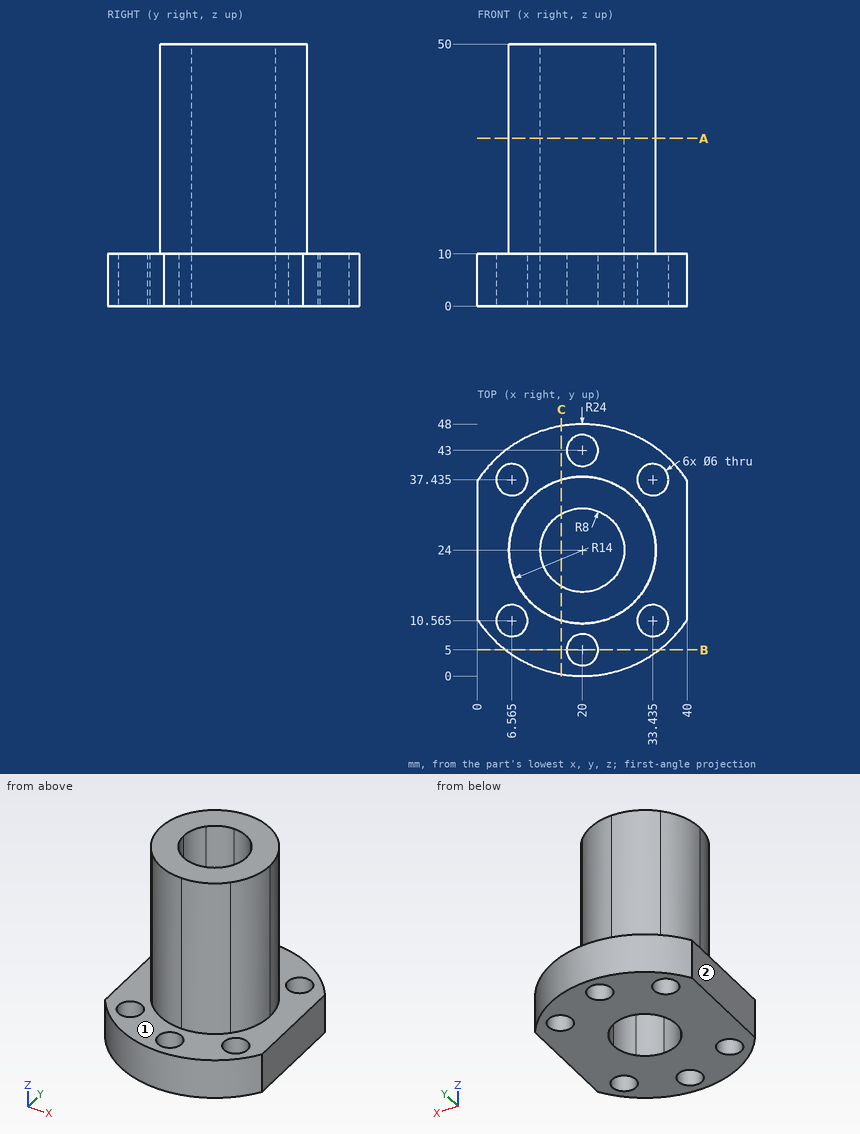
Source: three-view drawing plus pictorial views. Frame: mm from the lowest corner of the part. A direction names the side the tool comes from. Give positions to 0.01 mm unless a question says otherwise; leave off trailing zeros. Write each loop counter-clockwise with the first axis right and the second up, starting at its lowest first coordinate (ties: lowest second). Pieces come first, ordered by that corner, then holes. Notation, with made-up numbers: (24, -27.75) - (54, -27.75) arc R24 ccw to (54, 5.25) - close; hole circle Ø2 at (-30.75, 27). An arc over 180 degrees is marked (long way). Write item = value, one per line. Start each with the question number.
1. Ray query, L1, parallel to Y at x = 4, z = 3; L2, parallel to X at y = 11, z = 8; L3, parallel to Z at x = 3.5, y = 22. Return the intervals inside material, ascending.
2. Access query for the marked faces 1 and 2. Directions: +Z, -Z, +X, -X, +Y, -Y. A direction counts if a zero-diameter tool reaches every point of the face in a straight line with its end or side. Return the directions, or none.
3. Section query A-A, the plane z = 32. Output: boundary loops of the cut face in (x, y).
4. Section query B-B, the plane y = 5. Output: boundary loops of the cut face in (x, z), then the cut area to 3 significant figures.
5. Section query C-C, the plane x = 16. Output: boundary loops of the cut face in (y, z), then the cut area to 3 significant figures.
6. First-contact query: pin 1 Ø2 at (x, z) = (30.5, 21.5) entering from +Y; pin 2 Ø1.5 at (x, z) = (21.5, 30.5) entering from -Y; pin 3 Ø12 at (y, z) = (12.5, 35.5) entering from -X; pin 4 Ø5.5 at (x, y) = (33.44, 37.44) entering from +Z. Flat tips, straight axial feed; report the tip coordinate or a pass-through.
Check sheet entries:
q1.L1 = 6.11 to 9.01, 12.12 to 35.88, 38.99 to 41.89
q1.L2 = 0 to 3.6, 9.53 to 30.47, 36.4 to 40
q1.L3 = 0 to 10
q2.face_1 = +Z
q2.face_2 = +Z, -Z, -X, +Y, -Y
q3.outline = circle Ø28 at (20, 24); hole circle Ø16 at (20, 24)
q4.outline = (5.34, 0) - (17, 0) - (17, 10) - (5.34, 10) - close; (23, 0) - (34.66, 0) - (34.66, 10) - (23, 10) - close
q4.area = 233 mm2
q5.outline = (0.34, 0) - (17.07, 0) - (17.07, 50) - (10.58, 50) - (10.58, 10) - (0.34, 10) - close; (30.93, 0) - (47.66, 0) - (47.66, 10) - (37.42, 10) - (37.42, 50) - (30.93, 50) - close
q5.area = 854 mm2
q6.pin_1 = 34.28
q6.pin_2 = 10.02
q6.pin_3 = 7.13
q6.pin_4 = through
